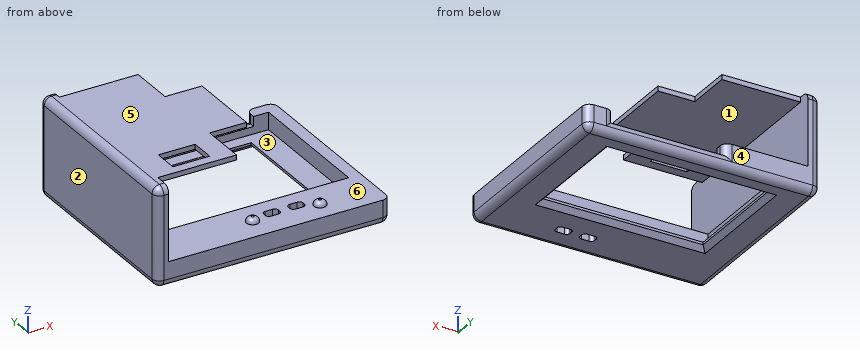
Autodesk Inventor part; units mm, degrees
ref_plane "YZ Plane" through (0, 0, 0) normal (1, 0, 0) x (0, 1, 0)
ref_plane "XZ Plane" through (0, 0, 0) normal (0, 1, 0) x (-1, 0, 0)
ref_plane "XY Plane" through (0, 0, 0) normal (0, 0, 1) x (1, 0, 0)
sketch "Sketch1" plane through (0, 0, 0) normal (0, 0, 1) x (1, 0, 0)
  line L0 (0, 0) -> (95, 0)
  line L1 (95, 0) -> (95, 80)
  line L2 (95, 80) -> (0, 80)
  line L3 (0, 80) -> (0, 0)
  dimension "d0" = 95
  dimension "d1" = 80
extrude "Extrusion1" add sketch "Sketch1" along normal blind 10
sketch "Sketch2" plane through (0, 0, 10) normal (0, 0, 1) x (1, 0, 0)
  line L0 (0, 0) -> (5, 0)
  line L1 (5, 0) -> (5, 80)
  line L2 (5, 80) -> (0, 80)
  line L3 (0, 80) -> (0, 0)
  dimension "d4" = 5
  dimension "d5" = 80
extrude "Extrusion2" add sketch "Sketch2" along normal blind 30
sketch "Sketch3" plane through (5, 0, 10) normal (1, 0, 0) x (0, 0, -1)
  line L0 (-30, 80) -> (-30, 0)
  line L1 (-30, 7.5) -> (-28, 7.5)
  line L2 (-28, 7.5) -> (-28, 75)
  line L3 (-28, 75) -> (-30, 75)
  line L4 (-30, 75) -> (-30, 7.5)
  point P0 (10, 0)
  dimension "d8" = 2
  dimension "d9" = 67.5
extrude "Extrusion3" add sketch "Sketch3" along normal blind 47
sketch "Sketch4" plane through (52, 0, 10) normal (1, 0, 0) x (0, 0, -1)
  line L0 (-28, 75) -> (-28, 7.5)
  line L1 (-28, 75) -> (-30, 75)
  line L2 (-30, 75) -> (-30, 56.5)
  line L3 (-30, 56.5) -> (-28, 56.5)
  line L4 (-28, 56.5) -> (-28, 75)
  line L5 (-28, 7.5) -> (-30, 7.5)
  line L6 (-30, 7.5) -> (-30, 26)
  line L7 (-30, 26) -> (-28, 26)
  line L8 (-28, 26) -> (-28, 7.5)
  point P0 (10, 0)
  dimension "d12" = 2
  dimension "d13" = 18.5
  dimension "d14" = 2
  dimension "d15" = 18.5
extrude "Extrusion4" cut sketch "Sketch4" against normal blind 15
sketch "Sketch5" plane through (0, 0, 40) normal (0, 0, 1) x (1, 0, 0)
  line L0 (28.5, 11.5) -> (13.5, 11.5)
  line L1 (13.5, 11.5) -> (13.5, 21.5)
  line L2 (13.5, 21.5) -> (28.5, 21.5)
  line L3 (28.5, 21.5) -> (28.5, 11.5)
  point P0 (0, 0)
  dimension "d18" = 15
  dimension "d19" = 10
extrude "Extrusion5" cut sketch "Sketch5" against normal blind 2
sketch "Sketch6" plane through (0, 0, 0) normal (0, 0, -1) x (-1, 0, 0)
  line L0 (-80, 70) -> (-15, 70)
  line L1 (-15, 70) -> (-15, 25)
  line L2 (-15, 25) -> (-80, 25)
  line L3 (-80, 25) -> (-80, 70)
  line L4 (0, 80) -> (0, 0)
  line L5 (-95, 80) -> (0, 80)
  dimension "d22" = 65
  dimension "d23" = 45
  dimension "d24" = 15
  dimension "d25" = 10
extrude "Extrusion6" cut sketch "Sketch6" against normal blind 10
sketch "Sketch7" plane through (0, 0, 0) normal (0, 0, -1) x (-1, 0, 0)
  point P0 (0, 0)
sketch "Sketch8" plane through (0, 0, 10) normal (0, 0, 1) x (1, 0, 0)
  line L0 (90, 20) -> (10, 20)
  line L1 (10, 20) -> (10, 75)
  line L2 (10, 75) -> (90, 75)
  line L3 (90, 75) -> (90, 20)
  point P0 (0, 0)
  dimension "d28" = 80
  dimension "d29" = 55
extrude "Extrusion7" cut sketch "Sketch8" against normal blind 7
sketch "Sketch9" plane through (0, 0, 10) normal (0, 0, 1) x (1, 0, 0)
  circle A0 centre (45, 10) radius 2.5
  line L0 (0, 0) -> (95, 0)
  line L1 (5, 80) -> (5, 0)
  dimension "d32" = 5
  dimension "d36" = 10
  dimension "d41" = 40
extrude "Extrusion8" add sketch "Sketch9" along normal blind 2
fillet "Fillet1" radius 2 1 edges at (42.5, 10, 12)
sketch "Sketch10" plane through (0, 0, 10) normal (0, 0, 1) x (1, 0, 0)
  circle A0 centre (71.5, 8.5) radius 2.5
  point P0 (0, 0)
  dimension "d37" = 5
extrude "Extrusion9" add sketch "Sketch10" along normal blind 2
fillet "Fillet2" radius 2 1 edges at (69, 8.5, 12)
fillet "Fillet3" radius 3 1 edges at (95, 0, 5)
fillet "Fillet4" radius 3 3 edges at (46, 0, 0) (94.1213, 0.8787, 0) (95, 41.5, 0)
fillet "Fillet5" radius 3 3 edges at (0, 41.5, 0) (0, 0.8787, 0.8787) (0, 0, 21.5)
fillet "Fillet6" radius 3 5 edges at (47.5, 80, 0) (0.8787, 80, 0.8787) (0, 80, 21.5) (94.1213, 80, 0.8787) (95, 80, 6.5)
fillet "Fillet7" radius 3 5 edges at (0, 40, 40) (0.8787, 0.8787, 40) (4, 0, 40) (0.8787, 79.1213, 40) (4, 80, 40)
chamfer "Chamfer1" distance 2 angle 45 1 edges at (47.5, 25, 0)
chamfer "Chamfer2" distance 2 angle 45 1 edges at (15, 47.5, 0)
chamfer "Chamfer3" distance 2 angle 45 1 edges at (80, 47.5, 0)
sketch "Sketch11" plane through (0, 0, 0) normal (0, 0, -1) x (-1, 0, 0)
  line L0 (-65.5, 10) -> (-62.5, 10)
  line L1 (-61, 11.5) -> (-61, 12.5)
  line L2 (-62.5, 14) -> (-65.5, 14)
  line L3 (-67, 12.5) -> (-67, 11.5)
  line L4 (-55.5, 10) -> (-52.5, 10)
  line L5 (-51, 11.5) -> (-51, 12.5)
  line L6 (-52.5, 14) -> (-55.5, 14)
  line L7 (-57, 12.5) -> (-57, 11.5)
  arc A0 (-51, 12.5) -> (-52.5, 14) centre (-52.5, 12.5) ccw
  arc A1 (-52.5, 10) -> (-51, 11.5) centre (-52.5, 11.5) ccw
  arc A2 (-57, 11.5) -> (-55.5, 10) centre (-55.5, 11.5) ccw
  arc A3 (-55.5, 14) -> (-57, 12.5) centre (-55.5, 12.5) ccw
  arc A4 (-61, 12.5) -> (-62.5, 14) centre (-62.5, 12.5) ccw
  arc A5 (-62.5, 10) -> (-61, 11.5) centre (-62.5, 11.5) ccw
  arc A6 (-67, 11.5) -> (-65.5, 10) centre (-65.5, 11.5) ccw
  arc A7 (-65.5, 14) -> (-67, 12.5) centre (-65.5, 12.5) ccw
  point P0 (0, 0)
  point P1 (-67, 10)
  point P2 (-61, 14)
  point P3 (-61, 10)
  point P4 (-67, 14)
  point P5 (-57, 10)
  point P6 (-51, 14)
  point P7 (-51, 10)
  point P8 (-57, 14)
  dimension "d56" = 6
  dimension "d57" = 4
  dimension "d60" = 1.5
extrude "Extrusion10" cut sketch "Sketch11" against normal blind 10
chamfer "Chamfer4" distance 2 angle 45 1 edges at (47.5, 70, 0)
sketch "Sketch12" plane through (0, 0, 10) normal (0, 0, 1) x (1, 0, 0)
  line L0 (92, 80) -> (5, 80)
  line L1 (10, 75) -> (90, 75)
  line L2 (38.911, 80) -> (83.911, 80)
  line L3 (83.911, 80) -> (83.911, 75)
  line L4 (83.911, 75) -> (38.911, 75)
  line L5 (38.911, 75) -> (38.911, 80)
  point P0 (0, 0)
  dimension "d64" = 45
extrude "Extrusion11" cut sketch "Sketch12" against normal blind 4
fillet "Fillet8" radius 3 1 edges at (61.411, 80, 6)
fillet "Fillet9" radius 3 2 edges at (83.911, 80, 4.5003) (83.911, 80, 8)
fillet "Fillet10" radius 3 2 edges at (38.911, 80, 4.5003) (38.911, 80, 8)
properties part number "case top"
Can you work these out from the model? Positions are in its coordinate system, mm. Face numbers are marked on the shaded views. A direction names the side the tool comes from. Coordinates: 2 decimals unless noted, no trailing zeros. Write each loop counter-clockwise with the first axis right and the second up, starting at its lowest first coordinate (ties: lowest second). Pieces come first, ordered by that corner, then holes. Notation, with made-up numbers: M -37.75,73.5 L -11.75,73.5 A29 cw -11.75,111.5 Z; hole C 85.25,44.5 d8. An arc over 180 degrees is marked long. Use one line per item in the form item = value.
Q1. For the marked faces 1, 2 and 3, which set-ups out of +Z, -Z, +X, -X, +Y, -Y let a thin tool reach every point of the face, with its end or its side?
Model answer:
face_1 = +X, +Y, -Y
face_2 = +Z, -Z, -X, +Y, -Y
face_3 = none
Q2. If we section it at B-B (z = 7.5): State how many separate pieces and enclosed holes the cut face has, then the cut area to 3 significant figures.
Model answer:
separate_pieces = 1
enclosed_holes = 2
area = 2,920 mm^2
Q3. If we section it at A-A (y = 37.5): Write out the boundary of the cut face in (x, z), then the cut area to 3 significant figures.
Model answer:
outline = M 0,3 A3 ccw 3,0 L 13,0 L 15,2 L 15,3 L 10,3 L 10,10 L 5,10 L 5,38 L 52,38 L 52,40 L 3,40 A3 ccw 0,37 Z; M 80,2 L 82,0 L 92,0 A3 ccw 95,3 L 95,10 L 90,10 L 90,3 L 80,3 Z
area = 429 mm^2
Q4. If we section it at D-D (z = 29): Write out the boundary of the cut face in (x, y), then the cut area to 3 significant figures.
Model answer:
outline = M 0,3 A3 ccw 3,0 L 5,0 L 5,80 L 3,80 A3 ccw 0,77 Z
area = 396 mm^2
Q5. If we section it at C-C (y = 16): Write out the boundary of the cut face in (x, z).
Model answer:
outline = M 0,3 A3 ccw 3,0 L 92,0 A3 ccw 95,3 L 95,10 L 5,10 L 5,38 L 13.5,38 L 13.5,40 L 3,40 A3 ccw 0,37 Z; M 28.5,38 L 37,38 L 37,40 L 28.5,40 Z
Q6. I need wall thicknesses on line 1 along X through (y, z) = (39.5, 31.5); line 2 along Z through (x, y) = (35.5, 69); line 3 along Z through (x, y) = (48, 17.5). Which ranges of each line are inside material? Lowest first, please. Write a range as from..to.
Model answer:
line_1 = 0..5
line_2 = 38..40
line_3 = 0..10
Q7. We'd pull the mould along Z, two halves only. Please class the marked faces 4, 5 and 6: +Z half, -Z half, draft (parallel to the pull), parting line (faces both ways), or undercut.
Model answer:
face_4 = draft
face_5 = +Z half
face_6 = undercut
Q8. For P1, Ø2, axis at x = 62, y = 76.5, coming from the +Z side; P2, Ø1.6, axis at y = 63, z = 39, coming from the +X side; P3, Ø14, axis at x = 27.5, y = 38.5, coming from the -Z side, each with a flat end and sliding along its axis, tell me the tip position at first contact or that it passes through.
Model answer:
P1 = 6
P2 = 37
P3 = 38
